from build123d import *

# Parameters (mm, degrees)
SKETCH1_R           = 6.4
SKETCH1_R_2         = 3
BOSS_EXTRUDE2_DEPTH = 65
SKETCH4_R           = 0.5
CUT_EXTRUDE1_DEPTH  = 7.4


with BuildPart() as part:
    # Sketch1 → Boss-Extrude2 (new body)
    with BuildSketch(Plane(origin=(0, 0, 0), x_dir=(1, 0, 0), z_dir=(0, 1, 0))):
        Circle(SKETCH1_R)
        Circle(SKETCH1_R_2, mode=Mode.SUBTRACT)
    extrude(amount=BOSS_EXTRUDE2_DEPTH)

    # Sketch2 → Revolve2 (revolve)
    with BuildSketch(Plane.XY):
        with BuildLine():
            Line((-6.4, 65), (-6.4, 66.5))
            Line((-6.4, 66.5), (-5.470962631, 71.377446189))
            ThreePointArc((-5.470962631, 71.377446189), (-4.867546878, 72.39824531), (-3.751870139, 72.8))
            Line((-3.751870139, 72.8), (0, 72.8))
            Line((0, 72.8), (0, 65))
            Line((0, 65), (-6.4, 65))
        make_face()
    revolve(axis=Axis((0, 72.8, 0), (0, -1, 0)))

    # Sketch4 → Cut-Extrude1 (cut, through all)
    with BuildSketch(Plane.XY):
        with Locations((0, 70)):
            Circle(SKETCH4_R)
    extrude(amount=-CUT_EXTRUDE1_DEPTH, mode=Mode.SUBTRACT)


solid = part.part
Verification items for the finished model (mm, model axes). A direction names the side the tool comes from. Give positions to 0.01 mm unless a question says otherwise; leave off trailing zeros. Order: outer loops, then holes, each group sorted by start corner. A loop starts at its lowest first (then second) coordinate and runs counter-clockwise, first axis right, second up. Notation, with made-up numbers: M -35.5,51 L 2.5,51 A25 ccw 2.5,85 Z; hole C 34,78 d11. An arc over 180 degrees is marked long. Use one line per item in the form item = value. Start each with the question number.
Q1. Mould release check, pull along Z, two halves, no side actions. Record for faces 1 (the conical face through (1.241, 70.057, 5.586)), 2 (the flat face through (0, 72.8, 0)), 3 (the flat face through (0, 65, 0)): +Z half, -Z half, draft (parallel to the pull), parting line (faces both ways), or undercut.
Q2. Go/stop test with flat-tipped pins: pin 1 Ø2 at (x, z) = (1, 1) entering from -Y; pin 2 Ø1 at (x, y) = (-1.5, 42.5) entering from -Z; pin 3 Ø3 at (x, y) = (-3, 21.5) entering from -Z. Record where each tip stops, or that it passes through.
Q3. Section check A-A (y = 33.5). Enter the section's corners in (x, z), then the cut area to 3 significant figures.
Q4. Scan lines: line 1 along Y through (x, z) = (0, -1.75); line 2 along Z through (x, y) = (0, 24); line 3 along Y through (x, z) = (1.5, -0.25). Record each from-to range of solid material in increasing order. Write a range as [from, to].
Q5. Access from +Z, -Z, +X, -X, +Y, -Y to the whole of each face (thin tool, end or side, straight path). Record for faces 4 (the flat face through (3, 0, 1)), 5 (the cylindrical face through (-3, 32, 0)).
Evaluation:
q1.face_1 = parting line
q1.face_2 = draft
q1.face_3 = undercut
q2.pin_1 = 65
q2.pin_2 = -6.32
q2.pin_3 = -6.22
q3.outline = C 0,0 d12.8; hole C 0,0 d6
q3.area = 100 mm2
q4.line_1 = [65, 69.5], [70.5, 72.8]
q4.line_2 = [-6.4, -3], [3, 6.4]
q4.line_3 = [65, 72.8]
q5.face_4 = +Z, -Z, +X, -X, -Y
q5.face_5 = -Y
